Geometry check sheet. Reference: drawing and pictorial views, mm from the part's lowest x, y, z. Give positions to 0.01 mm unless a question says otherwise; leave off trailing zeros. Write item = value, one per line. Start each with the question number.
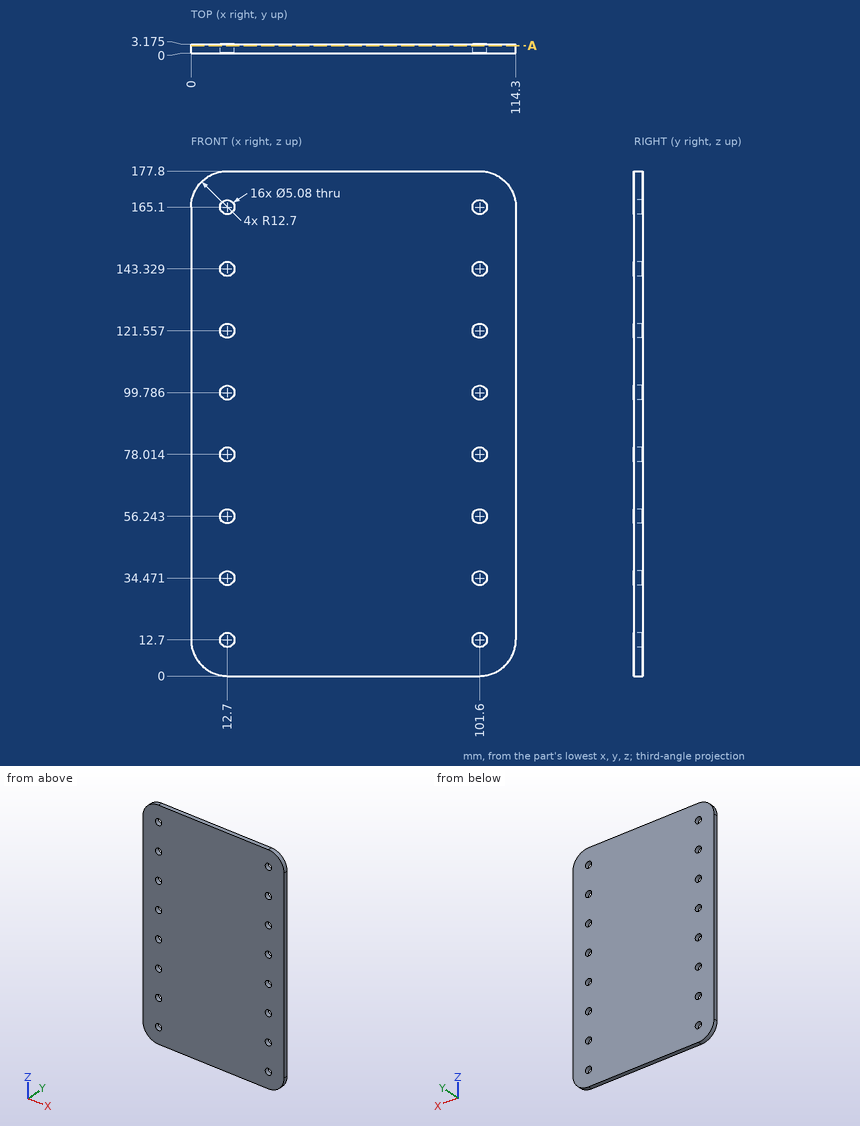
1) Thickness scan on line 1 (X direction, y = 0.35, z = 163.5); line 2 (Z direction, x = 108.5, y = 2.7). Record the ranges inside material, lowest first.
2) Depth check by flat-ended pin: pin 1 Ø6 at (x, z) = (101.6, 12.7) entering from +Y (3 decimals). Enter the tip coordinate at first touch or a pass-through.
3) Section check A-A (y = 2.6). Give the number of separate pieces and of enclosed holes in the cut face, plus the area to 3 significant figures.
Check result:
q1.line_1 = 0 to 10.73, 14.67 to 99.63, 103.57 to 114.3
q1.line_2 = 2.04 to 175.76
q2.pin_1 = 3.175
q3.separate_pieces = 1
q3.enclosed_holes = 16
q3.area = 19,900 mm2
